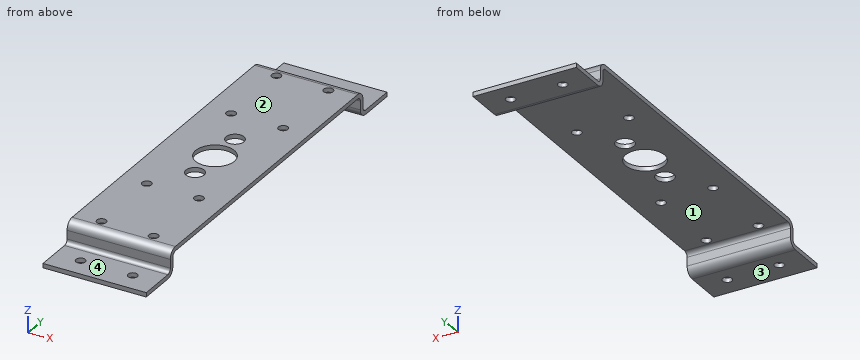
```python
from build123d import *

# Parameters (mm, degrees)
SALIENTE_EXTRUIR1_DEPTH   = 31.75
CONVERTIR_S_LIDO1_START   = -31.75
CONVERTIR_S_LIDO1_DEPTH   = 63.5
CONVERTIR_S_LIDO1_2_DEPTH = 63.5
CROQUIS7_R                = 2.8956
CROQUIS7_R_2              = 5.5499
CROQUIS7_R_3              = 11.9126
CORTAR_EXTRUIR1_DEPTH     = 132.88300309


# Read off the part's stored shape, not the designer's step: Convertir-Sólido1
with BuildPart() as part:
    # Croquis2 → Saliente-Extruir1 (new, symmetric)
    with BuildSketch(Plane(origin=(0, 0, 0), x_dir=(0, 0, -1), z_dir=(1, 0, 0))):
        Polygon((0, 101.6), (0, -101.6), (13.335, -101.6), (13.335, -127), (16.002, -127), (16.002, -98.933), (2.667, -98.933), (2.667, 98.933), (16.002, 98.933), (16.002, 127), (13.335, 127), (13.335, 101.6), align=None)
    extrude(amount=SALIENTE_EXTRUIR1_DEPTH, both=True)

    # Convertir-Sólido1 outline → Convertir-Sólido1 (cut)
    with BuildSketch(Plane.YZ.offset(CONVERTIR_S_LIDO1_START)):
        with BuildLine():
            Line((101.6, 0), (96.266, 0))
            ThreePointArc((96.266, 0), (100.037707571, -1.562292429), (101.6, -5.334))
            Line((101.6, -5.334), (101.6, 0))
        make_face()
        with BuildLine():
            Line((-101.6, 0), (-101.6, -5.334))
            ThreePointArc((-101.6, -5.334), (-100.037707571, -1.562292429), (-96.266, 0))
            Line((-96.266, 0), (-101.6, 0))
        make_face()
        with BuildLine():
            ThreePointArc((104.267, -16.002), (100.495292429, -14.439707571), (98.933, -10.668))
            Line((98.933, -10.668), (98.933, -16.002))
            Line((98.933, -16.002), (104.267, -16.002))
        make_face()
        with BuildLine():
            ThreePointArc((-98.933, -10.668), (-100.495292429, -14.439707571), (-104.267, -16.002))
            Line((-104.267, -16.002), (-98.933, -16.002))
            Line((-98.933, -16.002), (-98.933, -10.668))
        make_face()
    extrude(amount=CONVERTIR_S_LIDO1_DEPTH, mode=Mode.SUBTRACT)

    # Convertir-S_lido1 2 outline → Convertir-S_lido1 2 (add)
    with BuildSketch(Plane.YZ.offset(CONVERTIR_S_LIDO1_START)):
        with BuildLine():
            ThreePointArc((104.267, -13.335), (102.381146215, -12.553853785), (101.6, -10.668))
            Line((101.6, -10.668), (101.6, -13.335))
            Line((101.6, -13.335), (104.267, -13.335))
        make_face()
        with BuildLine():
            ThreePointArc((-101.6, -10.668), (-102.381146215, -12.553853785), (-104.267, -13.335))
            Line((-104.267, -13.335), (-101.6, -13.335))
            Line((-101.6, -13.335), (-101.6, -10.668))
        make_face()
        with BuildLine():
            Line((98.933, -2.667), (96.266, -2.667))
            ThreePointArc((96.266, -2.667), (98.151853785, -3.448146215), (98.933, -5.334))
            Line((98.933, -5.334), (98.933, -2.667))
        make_face()
        with BuildLine():
            Line((-98.933, -2.667), (-98.933, -5.334))
            ThreePointArc((-98.933, -5.334), (-98.151853785, -3.448146215), (-96.266, -2.667))
            Line((-96.266, -2.667), (-98.933, -2.667))
        make_face()
    extrude(amount=CONVERTIR_S_LIDO1_2_DEPTH)

    # Croquis7 → Cortar-Extruir1 (cut, through all)
    with BuildSketch(Plane.XY):
        with Locations((-16.002, -114.3)):
            Circle(CROQUIS7_R)
        with Locations((16.002, -114.3)):
            Circle(CROQUIS7_R)
        with Locations((-16.002, -92.202)):
            Circle(CROQUIS7_R)
        with Locations((16.002, -92.202)):
            Circle(CROQUIS7_R)
        with Locations((-16.002, -44.45)):
            Circle(CROQUIS7_R)
        with Locations((16.002, -44.45)):
            Circle(CROQUIS7_R)
        with Locations((0, -21.082)):
            Circle(CROQUIS7_R_2)
        Circle(CROQUIS7_R_3)
        with Locations(Location((0, 21.082, 0), (0, 0, 180))):
            Circle(CROQUIS7_R_2)
        with Locations(Location((16.002, 44.45, 0), (0, 0, 180))):
            Circle(CROQUIS7_R)
        with Locations(Location((-16.002, 44.45, 0), (0, 0, 180))):
            Circle(CROQUIS7_R)
        with Locations(Location((16.002, 92.202, 0), (0, 0, 180))):
            Circle(CROQUIS7_R)
        with Locations(Location((-16.002, 92.202, 0), (0, 0, 180))):
            Circle(CROQUIS7_R)
        with Locations(Location((16.002, 114.3, 0), (0, 0, 180))):
            Circle(CROQUIS7_R)
        with Locations(Location((-16.002, 114.3, 0), (0, 0, 180))):
            Circle(CROQUIS7_R)
    extrude(amount=-CORTAR_EXTRUIR1_DEPTH, mode=Mode.SUBTRACT)


solid = part.part
```
Geometry: final body of the model. Coordinates: model frame, mm. Face numbers are marked on the shaded views. A direction names the side the tool comes from. Coordinates: 2 decimals unless noted, no trailing zeros. Order: outer loops, then holes, each group sorted by start corner. A loop starts at its lowest first (then second) coordinate and runs counter-clockwise, first axis right, second up. Notation, with made-up numbers: (24, 67) -> (74, 67) arc R24 ccw to (74, 77) -> close; hole circle Ø10 at (-9, 34.25). An arc over 180 degrees is marked (long way). Answer in a Markdown table with one row per item.
Item 1: Section C-C on y = -44.45. Output: boundary loops of the cut face in (x, z).
Return value:
| item | result |
|---|---|
| outline | (-31.75, -2.67) -> (-18.9, -2.67) -> (-18.9, 0) -> (-31.75, 0) -> close; (-13.11, -2.67) -> (13.11, -2.67) -> (13.11, 0) -> (-13.11, 0) -> close; (18.9, -2.67) -> (31.75, -2.67) -> (31.75, 0) -> (18.9, 0) -> close |
Item 2: Access query for the marked faces 3 and 4. Directions: +Z, -Z, +X, -X, +Y, -Y. A direction counts if a zero-diameter tool reaches every point of the face in a straight line with its end or side. Return the directions, or none.
Return value:
| item | result |
|---|---|
| face 3 | -Z, +X, -X, +Y, -Y |
| face 4 | +Z, +X, -X, -Y |
Item 3: Contact query for flat-ended pins moving along their axis: P1, Ø12, axis at x = 19, y = 73.5, coming from the -Z side; P2, Ø6, axis at x = -1, z = -9, coming from the +Y side; P3, Ø2, axis at x = -13.5, z = -10.5, coming from the +Y side. Output: stop coordinate, or through.
Return value:
| item | result |
|---|---|
| P1 | stops at z = -2.67 |
| P2 | stops at y = 101.96 |
| P3 | stops at y = 101.73 |
Item 4: Ray query, L1, parallel to X at y = 44.45, z = -0.65; L2, parallel to Y at x = 24, z = -9.75; L3, parallel to Y at x = 0, z = -1.9. Return the intervals inside material, ascending.
Return value:
| item | result |
|---|---|
| L1 | x = -31.75 to -18.9, -13.11 to 13.11, 18.9 to 31.75 |
| L2 | y = -101.6 to -98.93, 98.93 to 101.6 |
| L3 | y = -100.35 to -26.63, -15.53 to -11.91, 11.91 to 15.53, 26.63 to 100.35 |
Item 5: Section B-B on x = 0. State how many separate pieces and enclosed holes the cut face has, plus the area to 3 significant figures.
Return value:
| item | result |
|---|---|
| separate pieces | 4 |
| enclosed holes | 0 |
| area | 607 mm² |
Item 6: Draft query along Y for the marked faces 1 and 2. Return one class per face: released by +Y, released by -Y, zero draft, split by the parting line, or undercut.
Return value:
| item | result |
|---|---|
| face 1 | undercut |
| face 2 | zero draft |
Item 7: Section A-A on y = 0. Output: boundary loops of the cut face in (x, z), plus the area to 3 significant figures.
Return value:
| item | result |
|---|---|
| outline | (-31.75, -2.67) -> (-11.91, -2.67) -> (-11.91, 0) -> (-31.75, 0) -> close; (11.91, -2.67) -> (31.75, -2.67) -> (31.75, 0) -> (11.91, 0) -> close |
| area | 106 mm² |
